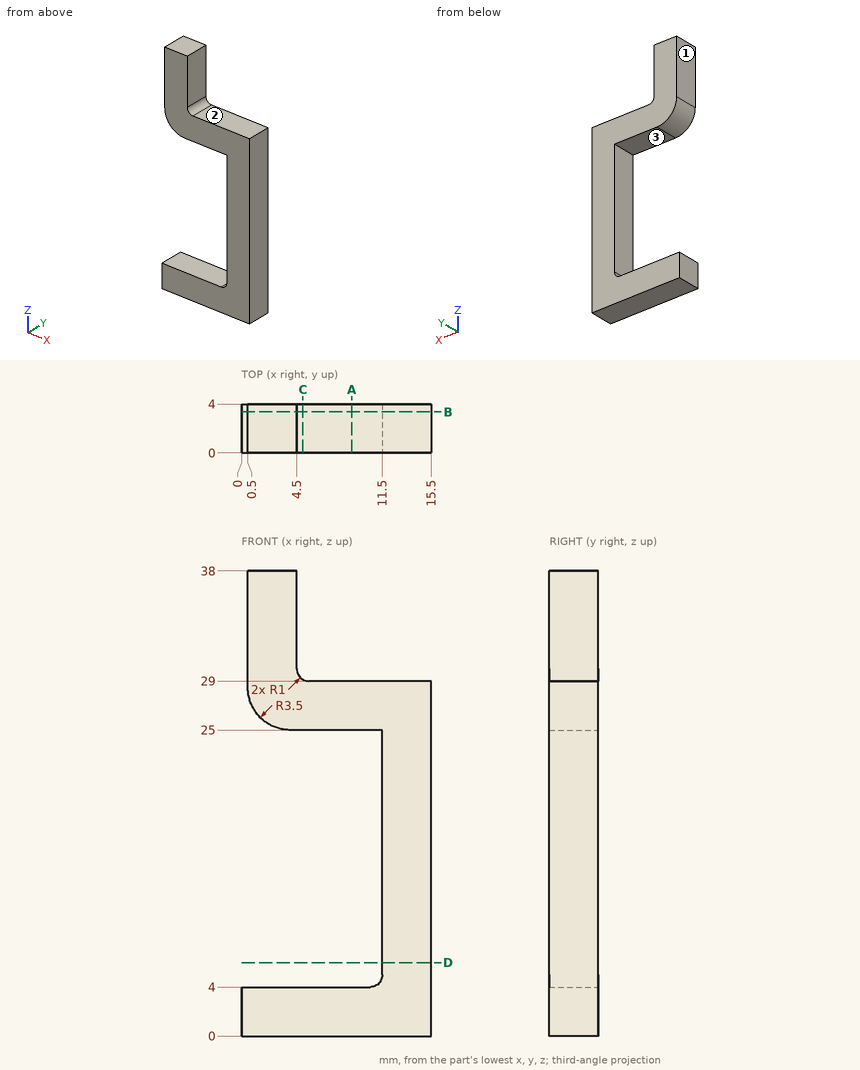
Geometry check sheet. Reference: drawing and pictorial views, mm from the part's lowest x, y, z. A direction names the side the tool comes from. Round coordinates to 2 decimals unless told otherwise and drop trailing zeros. Loops run counter-clockwise (first coordinate to the right, second up) from the corner with the lowest first, then second, coordinate; pieces in that order, holes last. Notation, with made-up numbers: (81, -29) - (91, -29) arc R15 ccw to (91, -9) - close; hole circle Ø8 at (35.25, -20). An arc over 180 degrees is marked (long way). Answer in a Markdown table with one row per item. Add a question column.
Q1. Tool access check on the marked faces 1, 2 and 3. Record the directions out of +Z, -Z, +X, -X, +Y, -Y that give a thin tool (end or side, any length) a straight path to the whole face; none if there is none.
Q2. Section check A-A on x = 9. Enter the section's corners in (y, z), plus the area to 3 significant figures.
Q3. Section check B-B on y = 3.35. Enter the section's corners in (x, z).
Q4. Section check D-D on z = 6. Enter the section's corners in (x, y).
Q5. Gauge pin test, flat ends, axial feed: pin 1 (2 mm diameter, centred on y = 1.5, z = 35, fed in from +X); pin 2 (2 mm diameter, centred on x = 6, y = 0.5, fed in from +Z); pin 3 (1.2 mm diameter, centred on x = 13, y = 1.5, fed in from +Z). Record the tip position at first contact, or that the pin passes through.
Q6. Section check C-C on x = 5. Enter the section's corners in (y, z), plus the area to 3 significant figures.
Q7. Material ranges on line 1 (Z direction, x = 7, y = 1.25); line 2 (Z direction, x = 4, y = 2.95); line 3 (X direction, y = 3.1, z = 16.5), recorded low to high.
Found:
| question | item | result |
|---|---|---|
| 1 | face 1 | +Z, -X, +Y, -Y |
| 1 | face 2 | +Z, +X, +Y, -Y |
| 1 | face 3 | -X, +Y, -Y |
| 2 | outline | (0, 0) - (4, 0) - (4, 4) - (0, 4) - close; (0, 25) - (4, 25) - (4, 29) - (0, 29) - close |
| 2 | area | 32.0 mm² |
| 3 | outline | (0, 0) - (15.5, 0) - (15.5, 29) - (5.5, 29) arc R1 cw to (4.5, 30) - (4.5, 38) - (0.5, 38) - (0.5, 28.5) arc R3.5 ccw to (4, 25) - (11.5, 25) - (11.5, 5) arc R1 cw to (10.5, 4) - (0, 4) - close |
| 4 | outline | (11.5, 0) - (15.5, 0) - (15.5, 4) - (11.5, 4) - close |
| 5 | pin 1 | stops at x = 4.5 |
| 5 | pin 2 | stops at z = 29.13 |
| 5 | pin 3 | stops at z = 29 |
| 6 | outline | (0, 0) - (4, 0) - (4, 4) - (0, 4) - close; (0, 25) - (4, 25) - (4, 29.13) - (0, 29.13) - close |
| 6 | area | 32.5 mm² |
| 7 | line 1 | z = 0 to 4, 25 to 29 |
| 7 | line 2 | z = 0 to 4, 25 to 38 |
| 7 | line 3 | x = 11.5 to 15.5 |
